Geometry: final body of the model. Coordinates: model frame, mm. A direction names the side the tool comes from. Give positions to 0.01 mm unless a question says otherwise; leave off trailing zeros. Write each loop counter-clockwise with the first axis right and the second up, starting at its lowest first coordinate (ties: lowest second). Pieces come first, ordered by that corner, then holes.
Q1. Section C-C (x = 0). Return the cut outline in (y, z), plus the area to 3 significant figures.
Q2. Reachability of faces 1 (the cylindrical face through (15.368, 11.832, -2.018)), 2 (the cylindrical face through (-24.513, 4.93, 0.195)) from +Z, -Z, +X, -X, +Y, -Y: full face, straight path, thin tool, end or side. Return the list, or none.
Q3. Mould query, pull axis X, two halves, no side actions, for faces 3 (the conical face through (-12.76, 23.03, -16.64)), 4 (the flat face through (-26, 10, 0)), 5 (the cylindrical face through (0.07, 4.93, -24.5)), 6 (the flat face through (1, 0, 17)). Classes: +X half, -X half, draft (parallel to the pull), parting line (faces both ways), or undercut.
Q4. Section A-A (z = 0). Return the cut outline in (x, y), plus the area to 3 significant figures.
Q5. Line query: line 1 (Z direction, x = -1, y = 2.75); line 2 (X direction, y = 16.5, z = 0); line 3 (X direction, y = 5, z = 0). Output: solid intervals per line, ascending.
Q6. Pin query (flat end, axial travel): pin 1 Ø2 at (y, z) = (3.5, 6) entering from +X; pin 2 Ø3 at (x, z) = (-25, 8.5) entering from +Y; pin 3 Ø12 at (x, y) = (-0.5, 20.5) entering from +Z. Return the tip coordinate at first contact, or that it passes through.
Q7. Section B-B (y = 9). Return the cut outline in (x, z), plus the area to 3 significant figures.
Q8. Section D-D (y = 21.5). Return the cut outline in (x, z), plus the area to 3 significant figures.
from build123d import *

# Parameters (mm, degrees)
SKETCH1_R           = 40
SKETCH1_R_2         = 15.5
BOSS_EXTRUDE1_DEPTH = 24
CHAMFER1_SIZE       = 20
SKETCH2_R           = 1.5
CUT_EXTRUDE1_DEPTH  = 10


with BuildPart() as part:
    # Sketch1 → Boss-Extrude1 (new body)
    with BuildSketch(Plane(origin=(0, 0, 0), x_dir=(1, 0, 0), z_dir=(0, 1, 0))):
        with Locations(Location((0, 0, 0), (0, 0, 270))):
            Circle(SKETCH1_R)
        with Locations(Location((0, 0, 0), (0, 0, 270))):
            Circle(SKETCH1_R_2, mode=Mode.SUBTRACT)
    extrude(amount=BOSS_EXTRUDE1_DEPTH)

    # Chamfer1
    chamfer1_edges = [part.edges().sort_by_distance(p)[0] for p in [
        (0, 24, -40),
    ]]
    chamfer(chamfer1_edges, length=CHAMFER1_SIZE)

    # Sketch2 → Cut-Extrude1 (cut)
    with BuildSketch(Plane.XZ):
        with Locations(Location((0, 26, 0), (0, 0, 270))):
            Circle(SKETCH2_R)
        with Locations(Location((26, 0, 0), (0, 0, 270))):
            Circle(SKETCH2_R)
        with Locations(Location((0, -26, 0), (0, 0, 270))):
            Circle(SKETCH2_R)
        with Locations(Location((-26, 0, 0), (0, 0, 270))):
            Circle(SKETCH2_R)
    extrude(amount=-CUT_EXTRUDE1_DEPTH, mode=Mode.SUBTRACT)


solid = part.part
Computed:
1. outline: (0, -40) - (4, -40) - (24, -20) - (24, -15.5) - (0, -15.5) - (0, -24.5) - (10, -24.5) - (10, -27.5) - (0, -27.5) - close; (0, 15.5) - (24, 15.5) - (24, 20) - (4, 40) - (0, 40) - (0, 27.5) - (10, 27.5) - (10, 24.5) - (0, 24.5) - close
1. area: 716 mm2
2. face 1: +Y, -Y
2. face 2: -Y
3. face 3: parting line
3. face 4: undercut
3. face 5: undercut
3. face 6: draft
4. outline: (-40, 0) - (-27.5, 0) - (-27.5, 10) - (-24.5, 10) - (-24.5, 0) - (-15.5, 0) - (-15.5, 24) - (-20, 24) - (-40, 4) - close; (15.5, 0) - (24.5, 0) - (24.5, 10) - (27.5, 10) - (27.5, 0) - (40, 0) - (40, 4) - (20, 24) - (15.5, 24) - close
4. area: 716 mm2
5. line 1: z = -39.99 to -27.12, -24.88 to -15.47, 15.47 to 24.88, 27.12 to 39.99
5. line 2: x = -27.5 to -15.5, 15.5 to 27.5
5. line 3: x = -39 to -27.5, -24.5 to -15.5, 15.5 to 24.5, 27.5 to 39
6. pin 1: stops at x = 39.69
6. pin 2: stops at y = 19.09
6. pin 3: stops at z = 29.5
7. outline: circle Ø70 at (0, 0); hole circle Ø3 at (-26, 0); hole circle Ø31 at (0, 0); hole circle Ø3 at (0, -26); hole circle Ø3 at (0, 26); hole circle Ø3 at (26, 0)
7. area: 3,070 mm2
8. outline: circle Ø45 at (0, 0); hole circle Ø31 at (0, 0)
8. area: 836 mm2
